Build history of the part. All positions in model axes, mm. A direction names the side the tool comes from. Round coordinates to 2 decimals unless told otherwise and drop trailing zeros. Write each loop counter-clockwise with the first axis right and the second up, starting at its lowest first coordinate (ties: lowest second). Pieces come first, ordered by that corner, then holes.
1) Flat gauge pins, fed straight in: pin 1 (14.5 mm diameter, centred on x = 0, y = 0, fed in from -Z); pin 2 (1.6 mm diameter, centred on x = -12, z = 1, fed in from -Y); pin 3 (1.5 mm diameter, centred on x = -15, y = 49, fed in from -Z); pin 4 (9.5 mm diameter, centred on x = 0, y = 0, fed in from +Z). Where does each tip first touch, or does it go through?
2) Pull direction Y, two halves, no side cores. Call faces 4 (the flat face through (0, 36, 0)), 5 (the flat face through (0, 145, -2)), 6 (the cylindrical face through (1.73, -7.81, 1.97)): +Y half, -Y half, draft (parallel to the pull), parting line (faces both ways), or undercut.
3) Saw through at C-C (z = -4.75). Write the cut outline in (x, y).
4) Saw through at D-D (x = -12). Write the cut outline in (y, z), plus the area to 3 significant figures.
5) Saw through at A-A (x = 0). Write the cut outline in (y, z), plus the area to 3 significant figures.
6) Wall check: probe 1 along X at (y, z) = (110, 1.25); probe 2 along Y at (x, z) = (-20, 0.25); probe 3 along Y at (x, z) = (11, 4). Give the ranges that are in metal, low to high.
7) Which spindle directions (+Z, -Z, +X, -X, +Y, -Y) get a long thin tool onto all of the face, cutting with end or side? Do faces 1 (the cylindrical face through (11.1, -10.5, 3.5)), 2 (the flat face through (10.6, -10.7, 2)), 3 (the flat face through (0, 105, -12)). Say none if no direction does.
8) Saw through at B-B (y = 140). Write the cut outline in (x, z).
from build123d import *

# Parameters (mm, degrees)
BOSS_EXTRUDE1_DEPTH = 5
SKETCH3_R           = 6
CUT_EXTRUDE2_DEPTH  = 36.707142143
SKETCH4_R           = 8
CUT_EXTRUDE3_DEPTH  = 4
SKETCH5_W           = 50
SKETCH5_H           = 120
BOSS_EXTRUDE2_DEPTH = 5
SKETCH6_R           = 1.75
CUT_EXTRUDE4_DEPTH  = 148.224318643
CUT_EXTRUDE5_DEPTH  = 2
SKETCH9_W           = 50
SKETCH9_H           = 40
BOSS_EXTRUDE3_DEPTH = 10
SKETCH10_W          = 50
SKETCH10_H          = 10
BOSS_EXTRUDE4_DEPTH = 15
SKETCH11_R          = 1.75
CUT_EXTRUDE6_DEPTH  = 148.901994577


with BuildPart() as part:
    # Sketch1 → Boss-Extrude1 (new body)
    with BuildSketch(Plane.XY):
        with BuildLine():
            Line((-25, 0), (-25, 25))
            Line((-25, 25), (25, 25))
            Line((25, 25), (25, 0))
            ThreePointArc((25, 0), (0, -25), (-25, 0))
        make_face()
    extrude(amount=BOSS_EXTRUDE1_DEPTH)

    # Sketch3 → Cut-Extrude2 (cut, through all)
    with BuildSketch(Plane(origin=(0, 0, 0), x_dir=(-1, 0, 0), z_dir=(0, 0, -1))):
        Circle(SKETCH3_R)
    extrude(amount=-CUT_EXTRUDE2_DEPTH, mode=Mode.SUBTRACT)

    # Sketch4 → Cut-Extrude3 (cut)
    with BuildSketch(Plane(origin=(0, 0, 0), x_dir=(-1, 0, 0), z_dir=(0, 0, -1))):
        Circle(SKETCH4_R)
    extrude(amount=-CUT_EXTRUDE3_DEPTH, mode=Mode.SUBTRACT)

    # Sketch5 → Boss-Extrude2 (add)
    with BuildSketch(Plane.XY):
        with Locations((0, 85)):
            Rectangle(SKETCH5_W, SKETCH5_H)
    extrude(amount=BOSS_EXTRUDE2_DEPTH)

    # Sketch6 → Cut-Extrude4 (cut, through all)
    with BuildSketch(Plane(origin=(0, 0, 0), x_dir=(-1, 0, 0), z_dir=(0, 0, -1))):
        with Locations((-12, -12)):
            Circle(SKETCH6_R)
        with Locations(Location((12, -12, 0), (0, 0, 180))):
            Circle(SKETCH6_R)
        with Locations((12, 12)):
            Circle(SKETCH6_R)
        with Locations(Location((-12, 12, 0), (0, 0, 180))):
            Circle(SKETCH6_R)
    extrude(amount=-CUT_EXTRUDE4_DEPTH, mode=Mode.SUBTRACT)

    # Sketch7 → Cut-Extrude5 (cut)
    with BuildSketch(Plane(origin=(0, 0, 0), x_dir=(-1, 0, 0), z_dir=(0, 0, -1))):
        Polygon((-8.709103466, -12), (-10.354551733, -9.15), (-13.645448267, -9.15), (-15.290896534, -12), (-13.645448267, -14.85), (-10.354551733, -14.85), align=None)
        Polygon((10.354551733, -14.85), (8.709103466, -12), (10.354551733, -9.15), (13.645448267, -9.15), (15.290896534, -12), (13.645448267, -14.85), align=None)
        Polygon((8.709103466, 12), (10.354551733, 9.15), (13.645448267, 9.15), (15.290896534, 12), (13.645448267, 14.85), (10.354551733, 14.85), align=None)
        Polygon((-10.354551733, 14.85), (-8.709103466, 12), (-10.354551733, 9.15), (-13.645448267, 9.15), (-15.290896534, 12), (-13.645448267, 14.85), align=None)
    extrude(amount=-CUT_EXTRUDE5_DEPTH, mode=Mode.SUBTRACT)

    # Sketch9 → Boss-Extrude3 (add)
    with BuildSketch(Plane(origin=(0, 0, 0), x_dir=(-1, 0, 0), z_dir=(0, 0, -1))):
        with Locations((0, 125)):
            Rectangle(SKETCH9_W, SKETCH9_H)
    extrude(amount=BOSS_EXTRUDE3_DEPTH)

    # Sketch10 → Boss-Extrude4 (add)
    with BuildSketch(Plane(origin=(0, 0, 0), x_dir=(-1, 0, 0), z_dir=(0, 0, -1))):
        with Locations((0, 100)):
            Rectangle(SKETCH10_W, SKETCH10_H)
    extrude(amount=BOSS_EXTRUDE4_DEPTH)

    # Sketch11 → Cut-Extrude6 (cut, through all)
    with BuildSketch(Plane(origin=(0, 0, -10), x_dir=(-1, 0, 0), z_dir=(0, 0, -1))):
        with Locations((-20, 140)):
            Circle(SKETCH11_R)
        with Locations(Location((20, 140, 0), (0, 0, 180))):
            Circle(SKETCH11_R)
        with Locations((20, 110)):
            Circle(SKETCH11_R)
        with Locations(Location((-20, 110, 0), (0, 0, 180))):
            Circle(SKETCH11_R)
    extrude(amount=-CUT_EXTRUDE6_DEPTH, mode=Mode.SUBTRACT)


solid = part.part
Evaluation:
1. pin 1: stops at z = 4
1. pin 2: stops at y = -22.35
1. pin 3: stops at z = 0
1. pin 4: passes through
2. face 4: draft
2. face 5: +Y half
2. face 6: undercut
3. outline: (-25, 95) - (25, 95) - (25, 145) - (-25, 145) - close; hole circle Ø3.5 at (-20, 110); hole circle Ø3.5 at (-20, 140); hole circle Ø3.5 at (20, 110); hole circle Ø3.5 at (20, 140)
4. outline: (-21.93, 0) - (-14.85, 0) - (-14.85, 2) - (-13.75, 2) - (-13.75, 5) - (-21.93, 5) - close; (-10.25, 2) - (-9.15, 2) - (-9.15, 0) - (9.15, 0) - (9.15, 2) - (10.25, 2) - (10.25, 5) - (-10.25, 5) - close; (13.75, 2) - (14.85, 2) - (14.85, 0) - (95, 0) - (95, -15) - (105, -15) - (105, -10) - (145, -10) - (145, 5) - (13.75, 5) - close
4. area: 1,340 mm2
5. outline: (-25, 0) - (-8, 0) - (-8, 4) - (-6, 4) - (-6, 5) - (-25, 5) - close; (6, 4) - (8, 4) - (8, 0) - (95, 0) - (95, -15) - (105, -15) - (105, -10) - (145, -10) - (145, 5) - (6, 5) - close
5. area: 1,320 mm2
6. probe 1: x = -25 to -21.75, -18.25 to 18.25, 21.75 to 25
6. probe 2: y = -15 to 108.25, 111.75 to 138.25, 141.75 to 145
6. probe 3: y = -22.45 to -13.44, -10.56 to 10.56, 13.44 to 145
7. face 1: +Z, -Z
7. face 2: -Z
7. face 3: -Z, +X, -X, +Y
8. outline: (-25, -10) - (-21.75, -10) - (-21.75, 5) - (-25, 5) - close; (-18.25, -10) - (18.25, -10) - (18.25, 5) - (-18.25, 5) - close; (21.75, -10) - (25, -10) - (25, 5) - (21.75, 5) - close
